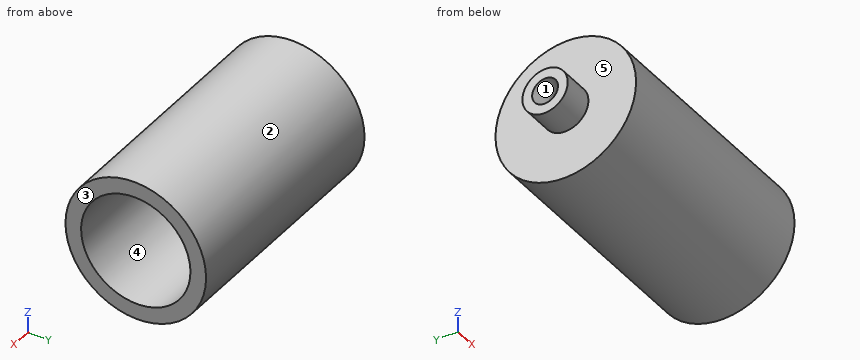
```python
from build123d import *


with BuildPart() as part:
    # Sketch1 → Revolve1 (revolve)
    with BuildSketch(Plane.XY, mode=Mode.PRIVATE) as revolve1_sk:
        with BuildLine():
            Line((6.35, 14.2875), (54.912326353, 14.2875))
            Line((54.912326353, 14.2875), (54.912326353, 11.1125))
            Line((54.912326353, 11.1125), (16.812326353, 11.1125))
            Line((16.812326353, 11.1125), (6.346118551, 2.330308893))
            ThreePointArc((6.346118551, 2.330308893), (4.992463664, 1.662760177), (3.483517422, 1.695685502))
            Line((3.483517422, 1.695685502), (0, 2.629091182))
            Line((0, 2.629091182), (0, 4.60375))
            Line((0, 4.60375), (6.35, 4.60375))
            Line((6.35, 4.60375), (6.35, 14.2875))
        make_face()
    revolve(revolve1_sk.sketch.rotate(Axis((0, 0, 0), (1, 0, 0)), 90), axis=Axis((0, 0, 0), (1, 0, 0)))


solid = part.part
```
Source: CAD feature listing. Evaluate the final solid. Frame: model axes, mm. Face numbers are marked on the shaded views. A direction names the side the tool comes from. Coordinates: 2 decimals unless noted, no trailing zeros. Order: outer loops, then holes, each group sorted by start corner. A loop starts at its lowest first (then second) coordinate and runs counter-clockwise, first axis right, second up. Notation, with made-up numbers: (65, 38.25) - (78, 38.25) arc R18 ccw to (78, 73.25) - close; hole circle Ø5 at (83, -31). An arc over 180 degrees is marked (long way). One line per item, written item: value.
1) Ray query, line 1 (Y direction, x = 42.5, z = 0); line 2 (X direction, y = -12, z = 2.5); line 3 (Y direction, x = 16, z = -0.5). Return the intervals inside material, ascending. Write a range as [from, to].
Computed values:
line 1: y = [-14.29, -11.11], [11.11, 14.29]
line 2: x = [6.35, 54.91]
line 3: y = [-14.28, -10.42], [10.42, 14.28]
2) Mould query, pull axis Y, two halves, no side actions, for the marked faces 1, 2 and 3. Classes: released by +Y, released by -Y, zero draft, split by the parting line, or undercut.
Computed values:
face 1: undercut
face 2: split by the parting line
face 3: zero draft
3) Cut plane D-D on x = 12.5. Output: boundary loops of the cut face in (y, z) (1 decimal), plus the area to 3 significant figures.
Computed values:
outline: circle Ø28.6 at (0, 0); hole circle Ø15 at (0, 0)
area: 465 mm^2
4) Contact query for flat-ended pins moving along their axis: pin 1 (3 mm diameter, centred on x = 24.5, y = 11, fed in from +Z); pin 2 (10 mm diameter, centred on x = 46.5, y = 9, fed in from -Z); pin 3 (5 mm diameter, centred on y = 9.5, z = -4, fed in from -X). Output: stop coordinate, or through.
Computed values:
pin 1: stops at z = 10.67
pin 2: stops at z = -13.72
pin 3: stops at x = 6.35
5) Reachability of the marked faces 4 and 5 from +Z, -Z, +X, -X, +Y, -Y: full face, straight path, thin tool, end or side. Return the list, or none.
Computed values:
face 4: +X
face 5: -X
6) Cut plane C-C on x = 26. Output: boundary loops of the cut face in (y, z) (1 decimal).
Computed values:
outline: circle Ø28.6 at (0, 0); hole circle Ø22.2 at (0, 0)
